Autodesk Inventor part; units mm, degrees
ref_plane "Work Plane1" through (0, 3, 0) normal (0, 1, 0) x (-1, 0, 0)
ref_plane "YZ Plane" through (0, 0, 0) normal (1, 0, 0) x (0, 1, 0)
ref_plane "XY Plane" through (0, 0, 0) normal (0, 0, 1) x (1, 0, 0)
sketch "Sketch1" plane through (0, 0, 0) normal (0, 1, 0) x (-1, 0, 0)
  line L0 (-51.65, 23.5) -> (51.65, 23.5)
  line L1 (54.65, 20.5) -> (54.65, -20.5)
  line L2 (51.65, -23.5) -> (-51.65, -23.5)
  line L3 (-54.65, -20.5) -> (-54.65, 20.5)
  circle A0 centre (-47.65, 16.5) radius 2.25
  circle A1 centre (47.65, 16.5) radius 2.25
  circle A2 centre (-47.65, 16.5) radius 26.75 construction
  circle A3 centre (-10.7, 16.5) radius 2.25
  circle A4 centre (-10.7, 16.5) radius 11.2 construction
  line L4 (-21.9, 16.5) -> (-21.9, 6.8604)
  line L5 (-20.9, 16.5) -> (-20.9, 6.8604)
  circle A5 centre (10.7, 16.5) radius 2.25
  circle A6 centre (10.7, 16.5) radius 11.2 construction
  line L6 (-0.5, 16.5) -> (-0.5, 5.694)
  line L7 (0.5, 16.5) -> (0.5, 5.694)
  circle A7 centre (47.65, 16.5) radius 26.75 construction
  line L8 (20.9, 16.5) -> (20.9, 5.8426)
  line L9 (21.9, 16.5) -> (21.9, 5.8426)
  arc A8 (-51.65, 23.5) -> (-54.65, 20.5) centre (-51.65, 20.5) ccw
  arc A9 (-54.65, -20.5) -> (-51.65, -23.5) centre (-51.65, -20.5) ccw
  arc A10 (54.65, 20.5) -> (51.65, 23.5) centre (51.65, 20.5) ccw
  arc A11 (51.65, -23.5) -> (54.65, -20.5) centre (51.65, -20.5) ccw
  line L10 (-84.9483, 16.5) -> (77.5332, 16.5) construction
  line L11 (-54.65, 0) -> (54.65, 0)
  line L12 (10.7, 30.5) -> (10.7, -33.5) construction
  circle A12 centre (10.7, -16.5) radius 2.25
  line L13 (5, -8.5) -> (18, -8.5) construction
  line L14 (3.7, -4.5) -> (3.7, -33.5) construction
  line L15 (-6.3, -4.5) -> (-6.3, -33.5) construction
  line L16 (-1.3, -33.5) -> (-1.3, -4.5) construction
  circle A13 centre (-1.3, -38.9) radius 2.25
  circle A14 centre (-1.3, -8.5) radius 2.25
  line L17 (-17.7373, -23.5) -> (14.2274, -23.5)
  line L18 (14.2274, -23.5) -> (14.2274, -45.3565)
  line L19 (14.2274, -45.3565) -> (-17.7373, -45.3565)
  line L20 (-17.7373, -45.3565) -> (-17.7373, -23.5)
  line L21 (-40.65, 5) -> (-30.65, 5)
  line L22 (-30.65, 5) -> (-30.65, -5)
  line L23 (-30.65, -5) -> (-40.65, -5)
  line L24 (-40.65, -5) -> (-40.65, 5)
  line L25 (-42.65, -7) -> (-28.65, -7)
  line L26 (-28.65, -7) -> (-28.65, 7)
  line L27 (-28.65, 7) -> (-42.65, 7)
  line L28 (-42.65, 7) -> (-42.65, -7)
  point P0 (0, 0)
  point P1 (-54.65, 23.5)
  point P2 (-54.65, -23.5)
  point P3 (0, 23.5)
  point P4 (-35.65, 5)
  point P5 (-30.65, 0)
  dimension "d5" = 53.5
  dimension "d12" = 53.5
  dimension "d1" = 4.5
  dimension "d2" = 7
  dimension "d3" = 4.5
  dimension "d4" = 7
  dimension "d6" = 4.5
  dimension "d7" = 22.4
  dimension "d8" = 1
  dimension "d9" = 4.5
  dimension "d10" = 22.4
  dimension "d11" = 1
  dimension "d13" = 1
  dimension "d14" = 3
  dimension "d23" = 16.5
  dimension "d24" = 7
  dimension "d27" = 8
  dimension "d28" = 7
  dimension "d29" = 10
  dimension "d30" = 5
  dimension "d31" = 4.5
  dimension "d32" = 4.5
  dimension "d33" = 30.4
  dimension "d38" = 0
  dimension "d40" = 10
  dimension "d41" = 10
  dimension "d43" = 2
  dimension "d47" = 12
ref_plane "Work Plane1" through (0, 3, 0) normal (0, 1, 0) x (-1, 0, 0)
sketch "Sketch3" plane through (0, 3, 0) normal (0, 1, 0) x (-1, 0, 0)
  circle A0 centre (-47.65, 16.5) radius 2.25
  circle A1 centre (-47.65, -16.5) radius 2.25
  circle A2 centre (-10.7, -16.5) radius 2.25
  circle A3 centre (10.7, -16.5) radius 2.25
  circle A4 centre (47.65, -16.5) radius 2.25
  circle A5 centre (47.65, 16.5) radius 2.25
  circle A6 centre (10.7, 16.5) radius 2.25
  circle A7 centre (-10.7, 16.5) radius 2.25
  line L0 (-54.65, 23.5) -> (-54.65, -23.5)
  line L1 (-54.65, -23.5) -> (54.65, -23.5)
  line L2 (54.65, 23.5) -> (-54.65, 23.5)
  line L3 (54.65, -23.5) -> (54.65, 23.5)
  line L4 (-40.65, 9.5) -> (-17.7, 9.5)
  line L5 (-17.7, 9.5) -> (-17.7, -23.5)
  line L6 (-40.65, -23.5) -> (-40.65, 9.5)
  line L7 (17.7, 9.5) -> (17.7, -23.5)
  line L8 (17.7, 9.5) -> (40.65, 9.5)
  line L9 (40.65, 9.5) -> (40.65, -23.5)
  circle A8 centre (-47.65, 16.5) radius 5.25
  circle A9 centre (47.65, 16.5) radius 5.25
  point P0 (0, 0)
  dimension "d66" = 7
  dimension "d67" = 7
  dimension "d68" = 7
  dimension "d69" = 7
  dimension "d71" = 7
  dimension "d72" = 7
  dimension "d73" = 7
  dimension "d74" = 7
  dimension "d75" = 7
  dimension "d76" = 7
  dimension "d80" = 3
  dimension "d81" = 3
extrude "Extrusion6" add sketch "Sketch3" against normal blind 3 contours L2 L3 L1 L9 L8 L7 L5 L4 L6 L0 | A8 | A9
fillet "Fillet2" radius 3 12 edges at (54.65, 1.5, 23.5) (54.65, 1.5, -23.5) (40.65, 1.5, -23.5) (40.65, 1.5, 9.5) (17.7, 1.5, 9.5) (17.7, 1.5, -23.5) (-17.7, 1.5, -23.5) (-17.7, 1.5, 9.5) (-40.65, 1.5, 9.5) (-40.65, 1.5, -23.5) (-54.65, 1.5, -23.5) (-54.65, 1.5, 23.5)
extrude "Extrusion7" add sketch "Sketch3" along normal blind 3 contours A8 | A9
mirror "Mirror3" about plane through (0, 0, 0) normal (0, 0, 1) of "Extrusion7"
properties part number "OuterBar"
Model file for the job. Use its own axes, mm. A direction names the side the tool comes from. Give positions to 0.01 mm unless a question says otherwise; leave off trailing zeros. Loops run counter-clockwise (first coordinate to the right, second up) from the corner with the lowest first, then second, coordinate; pieces in that order, holes last.
Item 1: Drop flat-ended pins along their axis: P1, Ø2.5, axis at x = 10.7, z = 16.5, coming from the +Y side; P2, Ø1.5, axis at x = 31, y = 1.5, coming from the -Z side; P3, Ø6, axis at x = -10.7, z = 16.5, coming from the +Y side. Give the stop position or say it passes through.
Check values:
P1: passes through
P2: stops at z = 9.5
P3: stops at y = 3
Item 2: Slice it at A-A (y = 4.75). Write the cut outline in (x, z).
Check values:
outline: circle Ø10.5 at (-47.65, -16.5); circle Ø10.5 at (-47.65, 16.5); circle Ø10.5 at (47.65, -16.5); circle Ø10.5 at (47.65, 16.5); hole circle Ø4.5 at (-47.65, -16.5); hole circle Ø4.5 at (-47.65, 16.5); hole circle Ø4.5 at (47.65, -16.5); hole circle Ø4.5 at (47.65, 16.5)
Item 3: Which spindle directions (+Z, -Z, +X, -X, +Y, -Y) get a long thin tool onto all of the face, cutting with end or side? Do faces 4 (the face through (-43.78, 4.48, -20.05)), 5 (the face through (41.51, 1.48, -22.6)), 6 (the face through (-53.79, 1.48, -22.6)). Say none if no direction does.
Check values:
face 4: +Y
face 5: -Z, +Y, -Y
face 6: -Z, -X, +Y, -Y
Item 4: Mould opens along X. For faces 1 (the face through (53.79, 1.48, 22.6)), 2 (the face through (48, 6, 14)), 3 (the face through (-18.56, 1.48, 8.6)) say: +X half, -X half, draft (parallel to the pull), parting line (faces both ways), or undercut.
Check values:
face 1: +X half
face 2: draft
face 3: undercut
Item 5: Drill centre lines: line 1 along Z through (x, y) = (-47.65, 4.45); line 2 along X through (y, z) = (0.6, 4.5); line 3 along Z through (x, y) = (10.7, 2.25). Where is each one in solid material? Low to high.
Check values:
line 1: z = -21.75 to -18.75, -14.25 to -11.25, 11.25 to 14.25, 18.75 to 21.75
line 2: x = -54.65 to -40.65, -17.7 to 17.7, 40.65 to 54.65
line 3: z = -23.5 to -18.75, -14.25 to 14.25, 18.75 to 23.5
Item 6: Slice it at B-B (z = -1.5). Write the cut outline in (x, y), plus the area to 3 significant figures.
Check values:
outline: (-54.65, 0) - (-40.65, 0) - (-40.65, 3) - (-54.65, 3) - close; (-17.7, 0) - (17.7, 0) - (17.7, 3) - (-17.7, 3) - close; (40.65, 0) - (54.65, 0) - (54.65, 3) - (40.65, 3) - close
area: 190 mm2
Item 7: Slice it at D-D (z = 16.5). Write the cut outline in (x, y), plus the area to 3 significant figures.
Check values:
outline: (-54.65, 0) - (-49.9, 0) - (-49.9, 6) - (-52.9, 6) - (-52.9, 3) - (-54.65, 3) - close; (-45.4, 0) - (-12.95, 0) - (-12.95, 3) - (-42.4, 3) - (-42.4, 6) - (-45.4, 6) - close; (-8.45, 0) - (8.45, 0) - (8.45, 3) - (-8.45, 3) - close; (12.95, 0) - (45.4, 0) - (45.4, 6) - (42.4, 6) - (42.4, 3) - (12.95, 3) - close; (49.9, 0) - (54.65, 0) - (54.65, 3) - (52.9, 3) - (52.9, 6) - (49.9, 6) - close
area: 310 mm2
Item 8: Slice it at C-C (x = 10.7). Write the cut outline in (y, z), plus the area to 3 significant figures.
Check values:
outline: (0, -23.5) - (3, -23.5) - (3, -18.75) - (0, -18.75) - close; (0, -14.25) - (3, -14.25) - (3, 14.25) - (0, 14.25) - close; (0, 18.75) - (3, 18.75) - (3, 23.5) - (0, 23.5) - close
area: 114 mm2
